Read the model definition and answer for the solid it produces. Units are mm, in the model's axes. Coordinates: 2 decimals unless noted, no trailing zeros. Order: outer loops, then holes, each group sorted by start corner. A loop starts at its lowest first (then second) coordinate and runs counter-clockwise, first axis right, second up. Notation, with made-up numbers: (29, 24) -> (50, 24) arc R19 cw to (50, 50) -> close; hole circle Ø6 at (-18, 48). An arc over 180 degrees is marked (long way). Use CSV: the item, a comma, the result in double quotes.
```python
from build123d import *

# Parameters (mm, degrees)
F0_R     = 25
F0_R_2   = 1.5
F1_DEPTH = 4
F2_SIZE  = 1
F3_R     = 2
F4_DEPTH = 4.001
F5_SIZE  = 1


with BuildPart() as f1:
    # F0 (on Front) → F1 (new body)
    with BuildSketch(Plane.XZ):
        Circle(F0_R)
        with Locations((-20, 0)):
            Circle(F0_R_2, mode=Mode.SUBTRACT)
        with Locations((20, 0)):
            Circle(F0_R_2, mode=Mode.SUBTRACT)
    extrude(amount=F1_DEPTH)

    # F2
    f2_edges = [f1.edges().sort_by_distance(p)[0] for p in [
        (-21.5, -4, 0),
        (18.5, -4, 0),
    ]]
    chamfer(f2_edges, length=F2_SIZE)

    # F3 (on face) → F4 (cut, through all)
    with BuildSketch(Plane.XZ.offset(4)):
        with Locations((0, 15)):
            Circle(F3_R)
        with Locations((0, -15)):
            Circle(F3_R)
    extrude(amount=-F4_DEPTH, mode=Mode.SUBTRACT)

    # F5
    f5_edges = [f1.edges().sort_by_distance(p)[0] for p in [
        (-2, 0, 15),
        (-2, 0, -15),
    ]]
    chamfer(f5_edges, length=F5_SIZE)


solid = f1.part
```
Item 1: Find section A-A, the plane z = -15. Give the vertices of the cut face in (x, y).
Return value:
outline,"(-20, -4) -> (-2, -4) -> (-2, -1) -> (-3, 0) -> (-20, 0) -> close; (2, -4) -> (20, -4) -> (20, 0) -> (3, 0) -> (2, -1) -> close"
Item 2: Find section B-B, the plane x = 0. Give the vertices of the cut face in (y, z), then the cut area to 3 significant figures.
Return value:
outline,"(-4, -25) -> (0, -25) -> (0, -18) -> (-1, -17) -> (-4, -17) -> close; (-4, -13) -> (-1, -13) -> (0, -12) -> (0, 12) -> (-1, 13) -> (-4, 13) -> close; (-4, 17) -> (-1, 17) -> (0, 18) -> (0, 25) -> (-4, 25) -> close"
area,"166 mm^2"
Item 3: Find section D-D, the plane z = -6. Give the vertices of the cut face in (x, y), then the cut area to 3 significant figures.
Return value:
outline,"(-24.27, -4) -> (24.27, -4) -> (24.27, 0) -> (-24.27, 0) -> close"
area,"194 mm^2"
Item 4: The mould has two halves that part along Z. Classify faces 1 (the cylindrical face through (0, -3, -13)), 2 (the cylindrical face through (23.846, -1.972, 7.509)), 3 (the flat face through (0, -4, 0)): +Z half, -Z half, draft (parallel to the pull), parting line (faces both ways), or undercut.
Return value:
face 1,"undercut"
face 2,"parting line"
face 3,"draft"
Item 5: Each of these flat-tipped pins is pushed along its axis until it touches: P1, Ø2, axis at y = -2.5, z = -11, coming from the -X side; P2, Ø2, axis at x = 13, y = -2.5, coming from the -Z side; P3, Ø4, axis at x = 20, z = 0, coming from the -Y side; P4, Ø6.5, axis at x = 0, z = 15, coming from the -Y side. Where does it stop, or does it pass through?
Return value:
P1,"stops at x = -22.91"
P2,"stops at z = -21.93"
P3,"stops at y = -3.5"
P4,"stops at y = -4"
Item 6: Find section C-C, the plane x = -20. Give the vertices of the cut face in (y, z), then the cut area to 3 significant figures.
Return value:
outline,"(-4, -15) -> (0, -15) -> (0, -1.5) -> (-3, -1.5) -> (-4, -2.5) -> close; (-4, 2.5) -> (-3, 1.5) -> (0, 1.5) -> (0, 15) -> (-4, 15) -> close"
area,"107 mm^2"
Item 7: Straight lines are drawn through the part: line 1 along Z through (x, y) = (0, -2.8); line 2 along Z through (x, y) = (-20, -2.3); line 3 along Z through (x, y) = (19, -3.2). For each, find the intervals that lie inside material, in ascending order.
Return value:
line 1,"z = -25 to -17, -13 to 13, 17 to 25"
line 2,"z = -15 to -1.5, 1.5 to 15"
line 3,"z = -16.25 to -1.37, 1.37 to 16.25"
